from build123d import *

# Parameters (mm, degrees)
F0_R          = 2.4010472057
F1_DEPTH      = 13.5382
F1_DEPTH_BACK = 13.5382
F2_R          = 3.2490620178
F3_DEPTH      = 2.54


# Not quite as in the source:
# - a pattern or mirror of a feature is missing from the dataset's text; its kind, count and spacing are read off the source's solid


with BuildPart() as f1:
    # F0 (on Top) → F1 (new body, two sides)
    with BuildSketch(Plane.XY) as f1_sk:
        Circle(F0_R)
    extrude(amount=F1_DEPTH)
    extrude(f1_sk.sketch, amount=-F1_DEPTH_BACK)

    # F2 (on face) → F3 (join)
    with BuildSketch(Plane.XY.offset(13.5382)):
        Circle(F2_R)
    f3 = extrude(amount=F3_DEPTH)

    # F3_copies: F3 across plane
    add(f3.mirror(Plane(origin=(0, 0, 0), x_dir=(-1, 0, 0), z_dir=(0, 0, -1))))


solid = f1.part
Could you check a few things on this model? Use its own coordinates, in mm. Give positions to 0.01 mm unless a question says otherwise; leave off trailing zeros. Order: outer loops, then holes, each group sorted by start corner. A loop starts at its lowest first (then second) coordinate and runs counter-clockwise, first axis right, second up. Notation, with made-up numbers: (-2, 38.5) - (10, 38.5) arc R18 ccw to (10, 69.5) - close; hole circle Ø10 at (-27.75, 70.5). An arc over 180 degrees is marked (long way). One line per question, with ' | ' between items. Start each with the question number.
Item 1: I'm going to push flat-ended pins straight in: pin 1 Ø3 at (y, z) = (0.5, 11) entering from +X; pin 2 Ø2 at (y, z) = (2, 1) entering from +X; pin 3 Ø3 at (x, z) = (1, 4.5) entering from +Y. Where does each tip first touch, or does it pass through?
Item 2: I want a section at A-A on y = 0. Write out the boundary of the cut face in (x, z), then the cut area to 3 significant figures.
Item 3: I want a section at C-C on z = -14. Write out the boundary of the cut face in (x, y).
Item 4: Thinking about a two-plate mould opening in Z: for faces 1 (the cylindrical face through (-1.77, 1.62, 0.19)), 2 (the flat face through (0, 0, -16.078)), 3 (the flat face through (0, 0, 16.078)), 4 (the cylindrical face through (3.001, -1.244, -14.79)), which applies, pulls with the +Z half, pulls with the -Z half, needs draft (parallel to the pull), parting line crosses it, or undercut?
Item 5: I want a section at D-D on z = 3.5. Write out the boundary of the cut face in (x, y), then the cut area to 3 significant figures.
Item 6: I need wall thicknesses on probe 1 along Z at (x, y) = (2.75, 1.5); probe 2 along X at (y, z) = (0.5, 11); probe 3 along Y at (x, z) = (0.75, -9). Which ranges of each line are inside material? Lowest first, please. Write a range as [from, to].
Verdict:
1) pin 1: x = 2.4 | pin 2: x = 2.18 | pin 3: y = 2.4
2) outline: (-3.25, -16.08) - (3.25, -16.08) - (3.25, -13.54) - (2.4, -13.54) - (2.4, 13.54) - (3.25, 13.54) - (3.25, 16.08) - (-3.25, 16.08) - (-3.25, 13.54) - (-2.4, 13.54) - (-2.4, -13.54) - (-3.25, -13.54) - close | area: 163 mm^2
3) outline: circle Ø6.5 at (0, 0)
4) face 1: undercut | face 2: pulls with the -Z half | face 3: pulls with the +Z half | face 4: needs draft
5) outline: circle Ø4.8 at (0, 0) | area: 18.1 mm^2
6) probe 1: [-16.08, -13.54], [13.54, 16.08] | probe 2: [-2.35, 2.35] | probe 3: [-2.28, 2.28]
